```python
from build123d import *

# Parameters (mm, degrees)
PAD014_DEPTH               = 1.28
PAD015_DEPTH               = 17
SKETCH018_W                = 82.4657333469
SKETCH018_H                = 103.1855755689
PAD016_DEPTH               = 8
PAD020_DEPTH               = 3
PAD020_MIRRORED008_2_DEPTH = 3
SKETCH026_R                = 1.5
POCKET002_DEPTH            = 4.301
MULTITRANSFORM004_FACE58_W = 3
MULTITRANSFORM004_FACE58_H = 6.72
PAD021_DEPTH               = 5
PAD021_FACE71_W            = 3
PAD021_FACE71_H            = 6.72
PAD022_DEPTH               = 4
SKETCH033_R                = 4.5
PAD029_DEPTH               = 3
SKETCH034_R                = 1.7
POCKET005_DEPTH            = 55.001


with BuildPart() as part:
    # Sketch016 → Pad014 (new body)
    with BuildSketch(Plane.XY):
        Polygon((-90, -56.28), (-90, 55), (0, 55), (0, 0), (0, -55), (-40, -55), (-40, -56.28), align=None)
    extrude(amount=-PAD014_DEPTH)

    # Sketch017 (on Face5 of Pad014) → Pad015 (join)
    with BuildSketch(Plane.XZ.offset(55)):
        with BuildLine():
            ThreePointArc((3.4899774441, -11.449751074), (11.8608235957, -7.2848139089), (6.0000000021, 0))
            Line((6.0000000021, 0), (0, 0))
            Line((-4, 0), (0, 0))
            Line((-4, -8), (-4, 0))
            Line((3.4899774441, -11.449751074), (-4, -8))
        make_face()
        with BuildLine():
            ThreePointArc((3.9023823037, -4.3), (3.3, -6), (3.9023823037, -7.7))
            Line((3.9023823037, -7.7), (8.0976176963, -7.7))
            ThreePointArc((8.0976176963, -7.7), (8.7, -6), (8.0976176963, -4.3))
            Line((3.9023823037, -4.3), (8.0976176963, -4.3))
        make_face(mode=Mode.SUBTRACT)
    extrude(amount=-PAD015_DEPTH)

    # Sketch018 → Pad016 (join)
    with BuildSketch(Plane.XY):
        with Locations((-44.2328666735, -1.4496544031)):
            Rectangle(SKETCH018_W, SKETCH018_H)
        Polygon((-5.4, -50.6424421875), (-83.0657333469, -50.6424421875), (-83.0657333469, -38.075158972), (-83.0657333469, -35.675158972), (-83.0657333469, 47.7431333814), (-5.4, 47.7431333814), (-5.4, -35.675159), (-5.4, -38.075157), align=None, mode=Mode.SUBTRACT)
    extrude(amount=-PAD016_DEPTH)

    # Sketch024 → Pad020 (join)
    with BuildSketch(Plane.XZ.offset(35)):
        Polygon((23, 0), (-3, 0), (-3, -8), (20, -8), align=None)
    pad020 = extrude(amount=PAD020_DEPTH)

    # Sketch024 Mirrored008 2 → Pad020 Mirrored008 2 (add)
    with BuildSketch(Plane(origin=(-10.8, -35, 0), x_dir=(-1, 0, 0), z_dir=(0, 1, 0))):
        Polygon((23, 0), (-3, 0), (-3, -8), (20, -8), align=None)
    pad020_mirrored008_2 = extrude(amount=-PAD020_MIRRORED008_2_DEPTH)

    # Mirrored009: Pad020, Pad020 Mirrored008 2 across XZ
    add(pad020.mirror(Plane.XZ))
    add(pad020_mirrored008_2.mirror(Plane.XZ))

    # Sketch026 (on Face40 of MultiTransform004) → Pocket002 (cut, through all)
    with BuildSketch(Plane.XY.offset(-7.7)):
        with Locations((6, -47.5)):
            Circle(SKETCH026_R)
    extrude(amount=-POCKET002_DEPTH, mode=Mode.SUBTRACT)

    # MultiTransform004 Face58 → Pad021 (add)
    with BuildSketch(Plane(origin=(-7.8, -36.5, -4.64), x_dir=(0, -1, 0), z_dir=(1, 0, 0))):
        Rectangle(MULTITRANSFORM004_FACE58_W, MULTITRANSFORM004_FACE58_H)
    extrude(amount=PAD021_DEPTH)

    # Pad021 Face71 → Pad022 (add)
    with BuildSketch(Plane(origin=(-7.8, 36.5, -4.64), x_dir=(0, -1, 0), z_dir=(1, 0, 0))):
        Rectangle(PAD021_FACE71_W, PAD021_FACE71_H)
    extrude(amount=PAD022_DEPTH)

    # Sketch033 → Pad029 (join)
    with BuildSketch(Plane.XZ.offset(-35)):
        with Locations((6, -6)):
            Circle(SKETCH033_R)
    extrude(amount=-PAD029_DEPTH)

    # Sketch034 → Pocket005 (cut, through all)
    with BuildSketch(Plane.XZ):
        with Locations((6, -6)):
            Circle(SKETCH034_R)
    extrude(amount=-POCKET005_DEPTH, mode=Mode.SUBTRACT)


solid = part.part
```
Check sheet for the modelled part. Datum: model origin and axes. Units: mm. A direction names the side the tool comes from. Round coordinates to 2 decimals unless told otherwise and drop trailing zeros. Order: outer loops, then holes, each group sorted by start corner. A loop starts at its lowest first (then second) coordinate and runs counter-clockwise, first axis right, second up. Notation, with made-up numbers: (-7.5, 20) - (2.5, 20) arc R30 cw to (2.5, 54) - close; hole circle Ø3 at (72.25, 20). An arc over 180 degrees is marked (long way). Answer as CSV lines item,"result". Start each with the question number.
1) Scan lines: probe 1 along Y at (x, z) = (6, -9.45); probe 2 along Y at (x, z) = (-9, -6); probe 3 along Z at (x, y) = (6, 35.65). Record each from-to range of solid material in increasing order.
2) Depth check by flat-ended pin: pin 1 (5.5 mm diameter, centred on x = -34, z = -6.5, fed in from -Y); pin 2 (3 mm diameter, centred on x = -8, y = -19, fed in from -Z); pin 3 (1.2 mm diameter, centred on x = 2, z = -10, fed in from +Y); pin 4 (2 mm diameter, centred on y = -32, z = -2, fed in from -X). Enter the tip coordinate at first touch or a pass-through.
3) Section check B-B (z = -6). Give the number of separate pieces and of enclosed holes in the cut face, then the cut area to 3 significant figures.
4) Section check C-C (y = 24). Record the cut outline in (x, z).
5) Tool access check on faces 1 (the face through (15, 37, -8)), 2 (the face through (-5.4, -44, -5)), 3 (the face through (4.6, -46.6, -7.7)). Record the directions out of +Z, -Z, +X, -X, +Y, -Y that give a thin tool (end or side, any length) a straight path to the whole face; none if there is none.
6) Section check D-D (x = -47). Record the cut outline in (y, z).
7) Section check A-A (x = 15). Record the cut outline in (y, z).
8) Draft check along X on faces 4 (the face through (21.479, -36.479, -4.056)), 5 (the face through (5.9, 36.5, -10.5)), 6 (the face through (16, -38, -4)), 7 (the face through (-32.04, 36.48, -4.69)). Enter one of: +X half, -X half, draft (parallel to the pull), parting line (faces both ways), or undercut.
Determined:
1,probe 1,"-55 to -49, -46 to -38, 35 to 38"
1,probe 2,"-53.04 to -50.64, -38 to -35, 35 to 38, 47.74 to 50.14"
1,probe 3,"-10.5 to -7.7, -4.3 to 0"
2,pin 1,"y = -53.04"
2,pin 2,"z = -1.28"
2,pin 3,"y = -38"
2,pin 4,"x = -90"
3,separate pieces,"2"
3,enclosed holes,"1"
3,area,"1,320 mm^2"
4,outline,"(-90, -1.28) - (-85.47, -1.28) - (-85.47, -8) - (-83.07, -8) - (-83.07, -1.28) - (-5.4, -1.28) - (-5.4, -8) - (-3, -8) - (-3, -1.28) - (0, -1.28) - (0, 0) - (-90, 0) - close"
5,face 1,"-Z, +X, +Y"
5,face 2,"-Z"
5,face 3,"-Y"
6,outline,"(-56.28, -1.28) - (-53.04, -1.28) - (-53.04, -8) - (-50.64, -8) - (-50.64, -1.28) - (47.74, -1.28) - (47.74, -8) - (50.14, -8) - (50.14, -1.28) - (55, -1.28) - (55, 0) - (-56.28, 0) - close"
7,outline,"(-38, -8) - (-35, -8) - (-35, 0) - (-38, 0) - close; (35, -8) - (38, -8) - (38, 0) - (35, 0) - close"
8,face 4,"+X half"
8,face 5,"parting line"
8,face 6,"draft"
8,face 7,"undercut"
